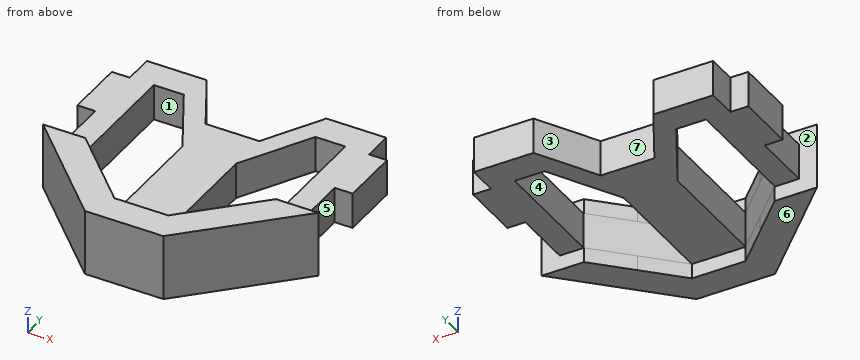
from build123d import *

# Parameters (mm, degrees)
BOSS_EXTRUDE1_DEPTH      = 6
BOSS_EXTRUDE2_DEPTH      = 2.5
BOSS_EXTRUDE2_DEPTH_BACK = 8.5


with BuildPart() as part:
    # Sketch1 → Boss-Extrude1 (new body)
    with BuildSketch(Plane.XY):
        Polygon((-20, -12.5), (-23, -12.5), (-6.55813284, -28.94186716), (6.55813284, -28.94186716), (23, -12.5), (20, -12.5), (20, -2.5), (23, -2.5), (23, 7.5), (20, 7.5), (20, 12.5), (10, 12.5), (4.487065029, 2.571710666), (-4.487065029, 2.571710666), (-10, 12.5), (-20, 12.5), (-20, 7.5), (-23, 7.5), (-23, -2.5), (-20, -2.5), align=None)
        Polygon((-16.000642854, -12.428289334), (-4.487065029, -23.94186716), (-4.487065029, -4.158644505), (-11.000642854, 7.571710666), (-16.000642854, 7.571710666), align=None, mode=Mode.SUBTRACT)
        Polygon((16.000642854, -12.428289334), (4.487065029, -23.94186716), (4.487065029, -4.158644505), (11.000642854, 7.571710666), (16.000642854, 7.571710666), align=None, mode=Mode.SUBTRACT)
    extrude(amount=BOSS_EXTRUDE1_DEPTH)

    # Sketch2 → Boss-Extrude2 (add, two sides: drawn at the far end of the back side and taken through both)
    with BuildSketch(Plane.XY.offset(6).offset(-BOSS_EXTRUDE2_DEPTH_BACK)):
        Polygon((-23, -12.5), (-6.55813284, -28.94186716), (6.55813284, -28.94186716), (23, -12.5), (15.928932188, -12.5), (10.243853941, -18.185078247), (4.487065029, -23.94186716), (-4.487065029, -23.94186716), (-10.243853941, -18.185078247), (-15.928932188, -12.5), align=None)
    extrude(amount=BOSS_EXTRUDE2_DEPTH + BOSS_EXTRUDE2_DEPTH_BACK)


solid = part.part
Could you check a few things on this model? Use its own coordinates, in mm. Face numbers are marked on the shaded views. A direction names the side the tool comes from. Give positions to 0.01 mm unless a question says otherwise; leave off trailing zeros. Order: outer loops, then holes, each group sorted by start corner. A loop starts at its lowest first (then second) coordinate and runs counter-clockwise, first axis right, second up. Notation, with made-up numbers: (20, 89.5) -> (61, 89.5) arc R23 cw to (61, 99.5) -> close; hole circle Ø4 at (40.25, 65.5). An arc over 180 degrees is marked (long way). Return JSON: item names as keys, results as strings.
1. Imagine slicing it at B-B on x = -19. List the corners of the cut face in (y, z) for me.
Answer list:
{"outline": "(-16.5, -2.5) -> (-12.5, -2.5) -> (-12.5, 0) -> (12.5, 0) -> (12.5, 6) -> (-12.5, 6) -> (-12.5, 8.5) -> (-16.5, 8.5) -> close"}
2. Thinking about a two-plate mould opening in Y: for the marked faces 4, 5, 6 and 7, which applies, pulls with the +Y half, pulls with the -Y half, needs draft (parallel to the pull), parting line crosses it, or undercut?
Answer list:
{"face 4": "undercut", "face 5": "undercut", "face 6": "needs draft", "face 7": "pulls with the +Y half"}
3. Imagine slicing it at A-A on z = 0.75. Give the number of separate pieces and of enclosed holes in the cut face, then the cut area to 3 significant figures.
Answer list:
{"separate pieces": "1", "enclosed holes": "2", "area": "885 mm2"}
4. I need wall thicknesses on line 1 (X direction, y = -4, z = 5.25); line 2 (X direction, y = 2.5, z = 2.25); line 3 (Y direction, x = -3.5, z = 1.5). Which ranges of each line are inside material? Lowest first, please. Write a range as from..to.
Answer list:
{"line 1": "x = -20..-16, -4.58..4.58, 16..20", "line 2": "x = -23..-16, -8.18..8.18, 16..23", "line 3": "y = -28.94..2.57"}
5. Imagine slicing it at C-C on y = -11. List the corners of the cut face in (x, z) for me, then the cut area to 3 significant figures.
Answer list:
{"outline": "(-20, 0) -> (-16, 0) -> (-16, 6) -> (-20, 6) -> close; (-4.49, 0) -> (4.49, 0) -> (4.49, 6) -> (-4.49, 6) -> close; (16, 0) -> (20, 0) -> (20, 6) -> (16, 6) -> close", "area": "102 mm2"}
6. For pin 1 Ø18 at (x, y) = (-1, 1.5) entering from +Z; pin 2 Ø2.5 at (x, z) = (-14.5, 3.5) entering from -Y; pin 3 Ø1.5 at (y, z) = (9.5, 2.5) entering from -X, each with a flat end and sliding along its axis, tell me the tip position at first contact or that it passes through.
Answer list:
{"pin 1": "stops at z = 6", "pin 2": "stops at y = -22.25", "pin 3": "stops at x = -20"}
7. Imagine slicing it at D-D on x = 12. List the corners of the cut face in (y, z) for me.
Answer list:
{"outline": "(-23.5, -2.5) -> (-16.43, -2.5) -> (-16.43, 8.5) -> (-23.5, 8.5) -> close; (7.57, 0) -> (12.5, 0) -> (12.5, 6) -> (7.57, 6) -> close"}
8. On a 3-axis mill with a long thin cutter (end or side, diameter ignored), from which of +Z, -Z, +X, -X, +Y, -Y can I reach the whole of each face in a straight line? I mean the marked faces 1, 2 and 3. Say none if no direction works.
Answer list:
{"face 1": "+Z, -Z", "face 2": "-X", "face 3": "+Z, -Z, +Y"}
